Can you work these out from the model? Positions are in its coordinate system, mm. Give positions to 0.01 mm unless a question says otherwise; leave off trailing zeros. Loops run counter-clockwise (first coordinate to the right, second up) from the corner with the lowest first, then second, coordinate; pieces in that order, holes last. Notation, with made-up numbers: (12.5, 9) - (30.5, 9) arc R9 cw to (30.5, 15) - close; hole circle Ø4 at (88, 78). An arc over 180 degrees is marked (long way). Answer in a Markdown table with one row per item.
from build123d import *

# Parameters (mm, degrees)
CROQUIS1_W              = 250
CROQUIS1_H              = 11
SALIENTE_EXTRUIR1_DEPTH = 6.35
CROQUIS2_W              = 250
CROQUIS2_H              = 3.175
SALIENTE_EXTRUIR2_DEPTH = 220
REDONDEO1_R             = 60
CROQUIS4_R              = 6.35
CORTAR_EXTRUIR1_DEPTH   = 11


with BuildPart() as part:
    # Croquis1 → Saliente-Extruir1 (new body)
    with BuildSketch(Plane(origin=(0, 0, 0), x_dir=(1, 0, 0), z_dir=(0, 1, 0))):
        with Locations((125, -0.308803141)):
            Rectangle(CROQUIS1_W, CROQUIS1_H)
    extrude(amount=SALIENTE_EXTRUIR1_DEPTH)

    # Croquis2 → Saliente-Extruir2 (add)
    with BuildSketch(Plane(origin=(0, 6.35, 0), x_dir=(1, 0, 0), z_dir=(0, 1, 0))):
        with Locations((125, 3.603696859)):
            Rectangle(CROQUIS2_W, CROQUIS2_H)
        with Locations((125, -4.221303141)):
            Rectangle(CROQUIS2_W, CROQUIS2_H)
    extrude(amount=SALIENTE_EXTRUIR2_DEPTH)

    # Redondeo1
    redondeo1_edges = [part.edges().sort_by_distance(p)[0] for p in [
        (250, 226.35, -3.603696859),
        (0, 226.35, -3.603696859),
        (0, 226.35, 4.221303141),
        (250, 226.35, 4.221303141),
    ]]
    fillet(redondeo1_edges, radius=REDONDEO1_R)

    # Croquis4 → Cortar-Extruir1 (cut)
    with BuildSketch(Plane(origin=(0, 0, -5.191196859), x_dir=(-1, 0, 0), z_dir=(0, 0, -1))):
        with Locations((-125, 166.35)):
            Circle(CROQUIS4_R)
    extrude(amount=-CORTAR_EXTRUIR1_DEPTH, mode=Mode.SUBTRACT)


solid = part.part
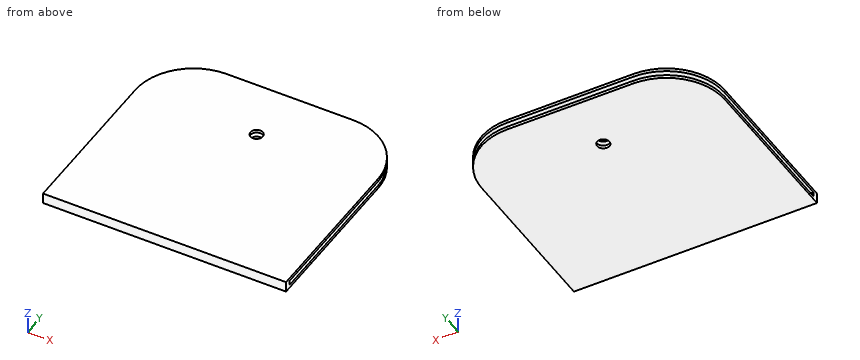
Q1. Imagine slicing it at A-A, the plane y = 50.5. Write out the boundary of the cut face in (x, z), and give its area (3 significant figures).
Checked values:
| item | result |
|---|---|
| outline | (0, -5.19) - (250, -5.19) - (250, -2.02) - (0, -2.02) - close; (0, 2.63) - (250, 2.63) - (250, 5.81) - (0, 5.81) - close |
| area | 1,590 mm² |
Q2. If I drill on line 1 (Z direction, x = 88, y = 108); line 2 (Y direction, x = 125, z = -3); line 3 (Y direction, x = 90, z = 0.25), over which ranges is the centre line in solid material (lowest first)? Write a range as [from, to].
Checked values:
| item | result |
|---|---|
| line 1 | z = [-5.19, -2.02], [2.63, 5.81] |
| line 2 | y = [0, 160], [172.7, 226.35] |
| line 3 | y = [0, 6.35] |
Q3. Imagine slicing it at C-C, the plane x = 162. Write out the boundary of the cut face in (y, z).
Checked values:
| item | result |
|---|---|
| outline | (0, -5.19) - (226.35, -5.19) - (226.35, -2.02) - (6.35, -2.02) - (6.35, 2.63) - (226.35, 2.63) - (226.35, 5.81) - (0, 5.81) - close |
Q4. For pin 1 (2.5 mm diameter, centred on x = 103, z = 0, fed in from +Y), with a flat end and sliding along its axis, tell me the tip position at first contact or that it passes through.
Checked values:
| item | result |
|---|---|
| pin 1 | stops at y = 6.35 |
Q5. Imagine slicing it at B-B, the plane x = 125. Write out the boundary of the cut face in (y, z), and give its area (3 significant figures).
Checked values:
| item | result |
|---|---|
| outline | (0, -5.19) - (160, -5.19) - (160, -2.02) - (6.35, -2.02) - (6.35, 2.63) - (160, 2.63) - (160, 5.81) - (0, 5.81) - close; (172.7, -5.19) - (226.35, -5.19) - (226.35, -2.02) - (172.7, -2.02) - close; (172.7, 2.63) - (226.35, 2.63) - (226.35, 5.81) - (172.7, 5.81) - close |
| area | 1,390 mm² |
Q6. Imagine slicing it at D-D, the plane y = 185.5. Write out the boundary of the cut face in (x, z), and give its area (3 significant figures).
Checked values:
| item | result |
|---|---|
| outline | (3.14, -5.19) - (246.86, -5.19) - (246.86, -2.02) - (3.14, -2.02) - close; (3.14, 2.63) - (246.86, 2.63) - (246.86, 5.81) - (3.14, 5.81) - close |
| area | 1,550 mm² |
